The listing builds one solid part. Answer for the finished solid, in the listing's coordinates (mm). A direction names the side the tool comes from. Round coordinates to 2 decimals unless told otherwise and drop trailing zeros. Loops run counter-clockwise (first coordinate to the right, second up) from the corner with the lowest first, then second, coordinate; pieces in that order, holes last. Notation, with made-up numbers: (61.5, 79.25) - (92.5, 79.25) arc R20 ccw to (92.5, 113.25) - close; hole circle Ø8 at (0, 37). An arc over 180 degrees is marked (long way). One line per item, written item: value.
```python
from build123d import *

# Parameters (mm, degrees)
F1_DEPTH = 25


with BuildPart() as f1:
    # F0 (on Top) → F1 (new body)
    with BuildSketch(Plane.XY):
        with BuildLine():
            ThreePointArc((-10.7, 0), (0, 10.7), (10.7, 0))
            Line((10.7, 0), (10.7, -20))
            ThreePointArc((10.7, -20), (12.1644660941, -23.5355339059), (15.7, -25))
            Line((15.7, -25), (105.7, -25))
            ThreePointArc((105.7, -25), (109.2355339059, -23.5355339059), (110.7, -20))
            Line((110.7, -20), (110.7, -10))
            Line((110.7, -10), (110.7, 0))
            ThreePointArc((110.7, 0), (109.2355339059, 3.5355339059), (105.7, 5))
            Line((105.7, 5), (95.7, 5))
            Line((95.7, 5), (95.7, -10))
            Line((95.7, -10), (70.5, -10))
            Line((70.5, -10), (70.5, -9))
            ThreePointArc((70.5, -9), (70.2071067812, -8.2928932188), (69.5, -8))
            Line((69.5, -8), (30.7, -8))
            add(Edge.make_bspline(
                [(25.7, -5), (25.7, -8), (30.7, -8)],
                knots=[0, 0, 0, 1.5707963268, 1.5707963268, 1.5707963268], degree=2, weights=[1, 0.7071067812, 1]))
            Line((25.7, -5), (25.7, 0))
            ThreePointArc((25.7, 0), (0, 25.7), (-25.7, 0))
            Line((-25.7, 0), (-25.7, -5))
            add(Edge.make_bspline(
                [(-30.7, -8), (-25.7, -8), (-25.7, -5)],
                knots=[4.7123889804, 4.7123889804, 4.7123889804, 6.2831853072, 6.2831853072, 6.2831853072], degree=2, weights=[1, 0.7071067812, 1]))
            Line((-30.7, -8), (-69.5, -8))
            ThreePointArc((-69.5, -8), (-70.2071067812, -8.2928932188), (-70.5, -9))
            Line((-70.5, -9), (-70.5, -10))
            Line((-70.5, -10), (-95.7, -10))
            Line((-95.7, -10), (-95.7, 5))
            Line((-95.7, 5), (-105.7, 5))
            ThreePointArc((-105.7, 5), (-109.2355339059, 3.5355339059), (-110.7, 0))
            Line((-110.7, 0), (-110.7, -10))
            Line((-110.7, -10), (-110.7, -20))
            ThreePointArc((-110.7, -20), (-109.2355339059, -23.5355339059), (-105.7, -25))
            Line((-105.7, -25), (-15.7, -25))
            ThreePointArc((-15.7, -25), (-12.1644660941, -23.5355339059), (-10.7, -20))
            Line((-10.7, -20), (-10.7, 0))
        make_face()
    extrude(amount=F1_DEPTH)


solid = f1.part
```
1) For faces 1 (the flat face through (-101, 5, 12)), 2 (the flat face through (101, 5, 12)), 3 (the flat face through (50, -8, 12)), 4 (the cylindrical face through (-12.2, -23.57, 12.32)), determine the directions among +Z, -Z, +X, -X, +Y, -Y from which every point of the face is accessible in a straight line to the end or side of a thin tool.
Final values:
face 1: +Z, -Z, -X, +Y
face 2: +Z, -Z, +X, +Y
face 3: +Z, -Z, +Y
face 4: +Z, -Z, -Y
2) A cutting plane is placed at A-A on y = -17. Give the vertices of the cut face in (x, z).
Final values:
outline: (-110.7, 0) - (-10.7, 0) - (-10.7, 25) - (-110.7, 25) - close; (10.7, 0) - (110.7, 0) - (110.7, 25) - (10.7, 25) - close
3) Each of these flat-tipped pins is pushed along its axis until it touches: pin 1 Ø1.5 at (y, z) = (15, 16.5) entering from +X; pin 2 Ø4 at (y, z) = (13, 6) entering from -X; pin 3 Ø11 at (x, z) = (100.5, 17.5) entering from +Y; pin 4 Ø5 at (x, y) = (22, -19.5) entering from -Z. Where does it stop, or does it pass through?
Final values:
pin 1: x = 21.39
pin 2: x = -23.23
pin 3: y = 5
pin 4: z = 0
4) For a pull along X with two mould halves and no side action, classify faces 5 (the flat face through (-25.7, -2, 12)), 6 (the cylindrical face through (-109.27, -23.5, 12.32)), 7 (the flat face through (-61, -25, 12)) as released by +X, released by -X, zero draft, split by the parting line, or undercut.
Final values:
face 5: undercut
face 6: released by -X
face 7: zero draft
5) A cutting plane is placed at B-B on x = 0. Give the vertices of the cut face in (y, z).
Final values:
outline: (10.7, 0) - (25.7, 0) - (25.7, 25) - (10.7, 25) - close
6) Consider L1, parallel to X at y = -2.5, z = 21.75; L2, parallel to X at y = -18.5, z = 22.5; L3, parallel to Y at x = -58, z = 19.75. Determine where each line is inside the solid, lowest interval first.
Final values:
L1: -110.7 to -95.7, -25.7 to -10.7, 10.7 to 25.7, 95.7 to 110.7
L2: -110.7 to -10.7, 10.7 to 110.7
L3: -25 to -8
7) A cutting plane is placed at C-C on x = -59. Give the vertices of the cut face in (y, z).
Final values:
outline: (-25, 0) - (-8, 0) - (-8, 25) - (-25, 25) - close
